Autodesk Inventor part; units mm, degrees
ref_plane "YZ Plane" through (0, 0, 0) normal (1, 0, 0) x (0, 1, 0)
ref_plane "XZ Plane" through (0, 0, 0) normal (0, 1, 0) x (-1, 0, 0)
ref_plane "XY Plane" through (0, 0, 0) normal (0, 0, 1) x (1, 0, 0)
sketch "スケッチ1" plane through (0, 0, 0) normal (0, 0, 1) x (1, 0, 0)
  circle A0 centre (0, 0) radius 4.25
  circle A1 centre (0, 0) radius 7
  dimension "d0" = 8.5
  dimension "d1" = 14
extrude "押し出し1" add sketch "スケッチ1" along normal mid plane 5
sketch "スケッチ2" plane through (0, 0, 2.5) normal (0, 0, 1) x (1, 0, 0)
  circle A0 centre (0, 0) radius 7
  circle A1 centre (0, 0) radius 2.15
  dimension "d9" = 4.3
extrude "押し出し2" add sketch "スケッチ2" along normal blind 2.5
chamfer "面取り2" distance 0.3 angle 45 3 edges at (-7, 0, 5) (-7, 0, -2.5) (-4.25, 0, -2.5)
properties part number "base40" material "ABS プラスチック"
Model file for the job. Use its own axes, mm. Coordinates: 2 decimals unless noted, no trailing zeros. Order: outer loops, then holes, each group sorted by start corner. A loop starts at its lowest first (then second) coordinate and runs counter-clockwise, first axis right, second up. Notation, with made-up numbers: M 78.5,73 L 95.5,73 A25 cw 95.5,98 Z; hole C -13.75,28 d6. An arc over 180 degrees is marked long. Return JSON: item names as keys, results as strings.
1. Drill centre lines: probe 1 along Y at (x, z) = (0, 4.15); probe 2 along Y at (x, z) = (0, 1.2); probe 3 along X at (y, z) = (1.5, 1.75). Where is each one in solid material? Low to high.
Ans:
{"probe 1": "-7 to -2.15, 2.15 to 7", "probe 2": "-7 to -4.25, 4.25 to 7", "probe 3": "-6.84 to -3.98, 3.98 to 6.84"}
2. Flat gauge pins, fed straight in: pin 1 (7 mm diameter, centred on x = -2, y = 1.5, fed in from -Z); pin 2 (5 mm diameter, centred on x = 0, y = 0, fed in from -Z). Where does each tip first touch, or does it go through?
Ans:
{"pin 1": "z = -2.5", "pin 2": "z = 2.5"}
3. Saw through at A-A (x = 0). Give the cut face in (y, z).
Ans:
{"outline": "M -7,-2.2 L -6.7,-2.5 L -4.55,-2.5 L -4.25,-2.2 L -4.25,2.5 L -2.15,2.5 L -2.15,5 L -6.7,5 L -7,4.7 Z; M 2.15,2.5 L 4.25,2.5 L 4.25,-2.2 L 4.55,-2.5 L 6.7,-2.5 L 7,-2.2 L 7,4.7 L 6.7,5 L 2.15,5 Z"}
4. Pull direction X, two halves, no side cores. Call faces 1 (the face through (2.285, -3.584, 0.117)), 2 (the face through (2, -2, 2.5)), 3 (the face through (6.466, 2.681, 1.202)), 4 (the face through (-2, 2, 5)): +X half, -X half, draft (parallel to the pull), parting line (faces both ways), or undercut.
Ans:
{"face 1": "undercut", "face 2": "undercut", "face 3": "parting line", "face 4": "draft"}
5. Saw through at C-C (z = 3.5). Give the cut face in (x, y).
Ans:
{"outline": "C 0,0 d14; hole C 0,0 d4.3"}
6. Saw through at D-D (z = -1). Give the cut face in (x, y).
Ans:
{"outline": "C 0,0 d14; hole C 0,0 d8.5"}
